Source: CAD feature listing. Evaluate the final solid. Frame: model axes, mm. Face numbers are marked on the shaded views. A direction names the side the tool comes from. Round coordinates to 2 decimals unless told otherwise and drop trailing zeros. Order: outer loops, then holes, each group sorted by start corner. A loop starts at its lowest first (then second) coordinate and runs counter-clockwise, first axis right, second up. Notation, with made-up numbers: M 32,-16 L 71,-16 A18 cw 71,-1 Z; hole C 25,-34 d10. An arc over 180 degrees is marked long. Use one line per item in the form item = value. Start each with the question number.
Q1. Section C-C (x = 0). Return the cut outline in (y, z).
Q2. Reachability of the marked faces 1, 2, 3 and 4 from +Z, -Z, +X, -X, +Y, -Y: full face, straight path, thin tool, end or side. Return the list, or none.
Q3. Contact query for flat-ended pins moving along their axis: pin 1 (3 mm diameter, centred on x = 7, y = 39, fed in from -Z); pin 2 (8 mm diameter, centred on x = 1, z = -37, fed in from -Y); pin 3 (2 mm diameter, centred on x = 12.5, y = 4.5, fed in from -Z). Output: stop coordinate, or through.
Q4. Section D-D (x = -12). Return the cut outline in (y, z).
Q5. Section A-A (z = 0). Return the cut outline in (x, y).
Q6. Material intervals for probe 1 along X at (y, z) = (0.5, 51); probe 2 along Z at (x, y) = (-19.5, 12.5), sorted ascending.
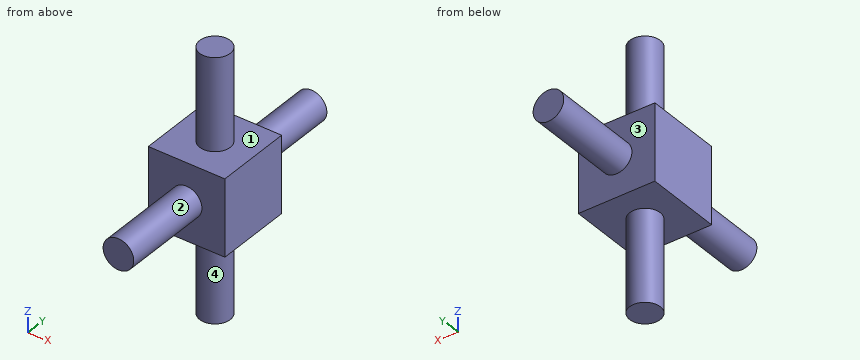
from build123d import *

# Parameters (mm, degrees)
F0_W          = 50
F0_H          = 50
F1_DEPTH      = 25
F1_DEPTH_BACK = 25
F2_R          = 10
F3_DEPTH      = 60
F4_R          = 10
F5_DEPTH      = 60
F6_R          = 10
F7_DEPTH      = 60
F8_R          = 10
F9_DEPTH      = 60


with BuildPart() as f1:
    # F0 (on Top) → F1 (new body, two sides)
    with BuildSketch(Plane.XY) as f1_sk:
        Rectangle(F0_W, F0_H)
    extrude(amount=F1_DEPTH)
    extrude(f1_sk.sketch, amount=-F1_DEPTH_BACK)

    # F2 (on face) → F3 (join)
    with BuildSketch(Plane.XZ.offset(25)):
        Circle(F2_R)
    extrude(amount=F3_DEPTH)

    # F4 (on face) → F5 (join)
    with BuildSketch(Plane(origin=(0, 0, -25), x_dir=(1, 0, 0), z_dir=(0, 0, -1))):
        Circle(F4_R)
    extrude(amount=F5_DEPTH)

    # F6 (on face) → F7 (join)
    with BuildSketch(Plane.XY.offset(25)):
        Circle(F6_R)
    extrude(amount=F7_DEPTH)

    # F8 (on face) → F9 (join)
    with BuildSketch(Plane(origin=(0, 25, 0), x_dir=(-1, 0, 0), z_dir=(0, 1, 0))):
        Circle(F8_R)
    extrude(amount=F9_DEPTH)


solid = f1.part
Results list:
q1.outline = M -85,-10 L -25,-10 L -25,-25 L -10,-25 L -10,-85 L 10,-85 L 10,-25 L 25,-25 L 25,-10 L 85,-10 L 85,10 L 25,10 L 25,25 L 10,25 L 10,85 L -10,85 L -10,25 L -25,25 L -25,10 L -85,10 Z
q2.face_1 = +Z
q2.face_2 = -Y
q2.face_3 = +Y
q2.face_4 = -Z
q3.pin_1 = -8.35
q3.pin_2 = -10
q3.pin_3 = -25
q4.outline = M -25,-25 L 25,-25 L 25,25 L -25,25 Z
q5.outline = M -25,-25 L -10,-25 L -10,-85 L 10,-85 L 10,-25 L 25,-25 L 25,25 L 10,25 L 10,85 L -10,85 L -10,25 L -25,25 Z
q6.probe_1 = -9.99 to 9.99
q6.probe_2 = -25 to 25
